Autodesk Inventor part; units mm, degrees
ref_plane "YZ Plane" through (0, 0, 0) normal (1, 0, 0) x (0, 1, 0)
ref_plane "XZ Plane" through (0, 0, 0) normal (0, 1, 0) x (-1, 0, 0)
ref_plane "XY Plane" through (0, 0, 0) normal (0, 0, 1) x (1, 0, 0)
sketch "Sketch1" plane through (0, 0, 0) normal (0, 1, 0) x (-1, 0, 0)
  line L0 (0, 0) -> (40, 0)
  line L1 (40, 0) -> (40, -40)
  line L2 (40, -40) -> (0, -40)
  line L3 (0, -40) -> (0, 0)
  dimension "d0" = 40
  dimension "d1" = 40
extrude "Extrusion1" add sketch "Sketch1" along normal blind 40
sketch "Sketch2" plane through (0, 40, 0) normal (0, 1, 0) x (1, 0, 0)
  circle A0 centre (-20, 20) radius 11.15
  line L0 (-40, 40) -> (-40, 0)
  line L1 (-40, 0) -> (0, 0)
  dimension "d4" = 22.3
  dimension "d5" = 20
  dimension "d6" = 20
extrude "Extrusion2" cut sketch "Sketch2" against normal blind 40
sketch "Sketch3" plane through (0, 0, 0) normal (1, 0, 0) x (0, 0, -1)
  line L0 (8.85, 25) -> (31.15, 25)
  line L1 (31.15, 25) -> (31.15, 15)
  line L2 (31.15, 15) -> (8.85, 15)
  line L3 (8.85, 15) -> (8.85, 25)
  line L4 (8.85, 25) -> (31.15, 15) construction
  line L5 (31.15, 25) -> (8.85, 15) construction
  line L6 (0, 0) -> (0, 40)
  line L7 (0, 40) -> (40, 40)
  point P0 (20, 20)
  dimension "d9" = 20
  dimension "d10" = 15
  dimension "d11" = 25
  dimension "d12" = 22.3
extrude "Extrusion3" cut sketch "Sketch3" against normal blind 20
fillet "Fillet1" radius 12.7 2 edges at (-20, 0, 0) (-20, 0, -40)
properties part number "YMount"
The model under review builds one solid part; all positions refer to its coordinate system, in mm. A direction names the side the tool comes from. Give positions to 0.01 mm unless a question says otherwise; leave off trailing zeros. Loops run counter-clockwise (first coordinate to the right, second up) from the corner with the lowest first, then second, coordinate; pieces in that order, holes last. Notation, with made-up numbers: (-8, 54) -> (25, 54) arc R36 ccw to (25, 90) -> close; hole circle Ø4 at (36, -13). An arc over 180 degrees is marked (long way). Answer as a JSON object with one key per item and string values. Group by question number.
Q1. Take a section at B-B (y = 32). Write out the cut boundary in (x, z).
Q2. Tool access review of faces 1 (the cylindrical face through (-34.13, 3.62, -36.18)), 2 (the flat face through (-10, 20, -8.85)), 3 (the cylindrical face through (-34.3, 3.62, -3.82)): name each direction out of +Z, -Z, +X, -X, +Y, -Y from which nothing blocks a thin tool from reaching the whole face with its end or side.
Q3. Draft analysis for pull direction Z (two halves, no side actions). For faces 4 (the flat face through (-4, 0, -20)), 5 (the flat face through (-5, 25, -20)), 6 (the cylindrical face through (-5.87, 3.62, -3.82)), state which applies: pulls with the +Z half, pulls with the -Z half, needs draft (parallel to the pull), parting line crosses it, or undercut.
Q4. Insertion check: pin 1 (12 mm diameter, centred on x = -29, y = 4.5, fed in from -Z); pin 2 (8 mm diameter, centred on x = -34, y = 4.5, fed in from +Z); pin 3 (6 mm diameter, centred on x = -30.5, z = -4, fed in from -Y). Each pin has a flat end and moves straight along its axis. Give the tip position at first contact, or say it passes through.
Q5. Take a section at D-D (z = -25). Write out the cut boundary in (x, y).
Q6. Take a section at A-A (z = -20). Write out the cut boundary in (x, y).
Q7. Take a section at C-C (y = 19.5). Write out the cut boundary in (x, z), plus the area to 3 significant figures.
Q8. Wall thickness on line 1 along X through (y, z) = (26, -20): over which ranges is the line inside the solid? List them lowest first.
Answer below:
{
 "1": {"outline": "(-40, -40) -> (0, -40) -> (0, 0) -> (-40, 0) -> close; hole circle Ø22.3 at (-20, -20)"},
 "2": {"face 1": "-Z, -X, -Y", "face 2": "+X", "face 3": "+Z, -X, -Y"},
 "3": {"face 4": "needs draft", "face 5": "undercut", "face 6": "pulls with the +Z half"},
 "4": {"pin 1": "stops at z = -39.81", "pin 2": "stops at z = -0.71", "pin 3": "stops at y = 1.35"},
 "5": {"outline": "(-40, 0) -> (-29.97, 0) -> (-29.97, 40) -> (-40, 40) -> close; (-10.03, 0) -> (0, 0) -> (0, 15) -> (-10.03, 15) -> close; (-10.03, 25) -> (0, 25) -> (0, 40) -> (-10.03, 40) -> close"},
 "6": {"outline": "(-40, 0) -> (-31.15, 0) -> (-31.15, 40) -> (-40, 40) -> close; (-8.85, 0) -> (0, 0) -> (0, 15) -> (-8.85, 15) -> close; (-8.85, 25) -> (0, 25) -> (0, 40) -> (-8.85, 40) -> close"},
 "7": {"outline": "(-40, -40) -> (0, -40) -> (0, -31.15) -> (-20, -31.15) arc R11.15 cw to (-20, -8.85) -> (0, -8.85) -> (0, 0) -> (-40, 0) -> close", "area": "959 mm2"},
 "8": {"line 1": "x = -40 to -31.15, -8.85 to 0"}
}
